For this review, take the finished solid that the model builds, in its own axes (mm). A direction names the side the tool comes from. Give positions to 0.01 mm unless a question says otherwise; leave off trailing zeros. Write each loop counter-clockwise with the first axis right and the second up, starting at its lowest first coordinate (ties: lowest second). Pieces come first, ordered by that corner, then holes.
1) Draft analysis for pull direction X (two halves, no side actions). For faces 3 (the face through (3.755, 61.625, 11.923)), 4 (the face through (0, 124, 0)), 5 (the face through (-5.4, 0, -0.2)), state which applies: pulls with the +X half, pulls with the -X half, needs draft (parallel to the pull), parting line crosses it, or undercut.
2) We need section C-C on y = 112. Give the boundary of the cut face in (x, z).
3) For P1, Ø4, axis at x = 0, z = -7.5, coming from the -Y side; P2, Ø1.5, axis at y = 64.5, z = 7, coming from the -X side; P3, Ø4, axis at y = 89.5, z = -3.5, coming from the -X side, all flat-tipped, find the tip position at first contact; note any pin that passes through.
4) Machinability: for faces 1 (the face through (-4.88, -1.97, -1.08)), 2 (the face through (3, 125, 8.2)), which of the approach directions +Z, -Z, +X, -X, +Y, -Y give a long, thin tool a straight path to every point of the face, cutting with its end or side? Answer none if there is none.
5) Wall thickness on line 1 along Y through (x, z) = (9, -3.5); line 2 along Y through (x, z) = (2.5, 4.5); line 3 along Z through (x, y) = (-0.75, 16.5): over which ranges is each line inside the solid? List them lowest first.
from build123d import *

# Parameters (mm, degrees)
SKETCH_1_R          = 12.5
EXTRUDE_1_DEPTH     = 125
SKETCH_2_R          = 5
EXTRUDE_2_DEPTH     = 5
FILLET_1_R          = 1
SKETCH_3_R          = 8.5
CUT_EXTRUDE_1_DEPTH = 1
FILLET_2_R          = 1


with BuildPart() as part:
    # 草图1 → 凸台-拉伸1 (new body)
    with BuildSketch(Plane(origin=(0, 0, 0), x_dir=(1, 0, 0), z_dir=(0, 1, 0))):
        with Locations(Location((0, 0, 0), (0, 0, 270))):
            Circle(SKETCH_1_R)
    extrude(amount=EXTRUDE_1_DEPTH)

    # 草图2 → 凸台-拉伸2 (add)
    with BuildSketch(Plane(origin=(0, 0, 0), x_dir=(1, 0, 0), z_dir=(0, 1, 0))):
        with Locations(Location((0, 0, 0), (0, 0, 270))):
            Circle(SKETCH_2_R)
    extrude(amount=-EXTRUDE_2_DEPTH)

    # 圆角1
    fillet_1_edges = [part.edges().sort_by_distance(p)[0] for p in [
        (0, -5, -5),
    ]]
    fillet(fillet_1_edges, radius=FILLET_1_R)

    # 草图3 → 切除-拉伸1 (cut)
    with BuildSketch(Plane(origin=(0, 125, 0), x_dir=(1, 0, 0), z_dir=(0, 1, 0))):
        with Locations(Location((0, 0, 0), (0, 0, 270))):
            Circle(SKETCH_3_R)
    extrude(amount=-CUT_EXTRUDE_1_DEPTH, mode=Mode.SUBTRACT)

    # 圆角2
    fillet_2_edges = [part.edges().sort_by_distance(p)[0] for p in [
        (0, 124, -8.5),
    ]]
    fillet(fillet_2_edges, radius=FILLET_2_R - 0.0001)  # a hair under: the kernel refuses the full size


solid = part.part
Results list:
1. face 3: parting line crosses it
1. face 4: undercut
1. face 5: needs draft
2. outline: circle Ø25 at (0, 0)
3. P1: stops at y = 0
3. P2: stops at x = -10.83
3. P3: stops at x = -12.41
4. face 1: -Y
4. face 2: +Z, -Z, +X, -X, +Y
5. line 1: y = 0 to 125
5. line 2: y = 0 to 124
5. line 3: z = -12.48 to 12.48
